```python
from build123d import *

# Parameters (mm, degrees)
F1_DEPTH = 38
F3_DEPTH = 25


with BuildPart() as f1:
    # F0 (on Right) → F1 (new body)
    with BuildSketch(Plane.YZ):
        Polygon((15, 19), (15, 20), (15, 24), (11, 24), (11, 15), (11, 6), (15, 6), (15, 10), (15, 11), (21.5, 11), (21.5, 8), (23.5, 8), (23.5, 15), (23.5, 22), (21.5, 22), (21.5, 19), align=None)
    extrude(amount=F1_DEPTH)

    # F2 (on face) → F3 (cut)
    with BuildSketch(Plane(origin=(0, 23.5, 0), x_dir=(-1, 0, 0), z_dir=(0, 1, 0))):
        with BuildLine():
            ThreePointArc((-17.35, 15), (-17.833274, 16.166726), (-19, 16.65))
            Line((-19, 16.65), (-19, 13.35))
            ThreePointArc((-19, 13.35), (-17.833274, 13.833274), (-17.35, 15))
        make_face()
        with BuildLine():
            Line((-19, 13.35), (-19, 16.65))
            ThreePointArc((-19, 16.65), (-20.65, 15), (-19, 13.35))
        make_face()
    extrude(amount=-F3_DEPTH, mode=Mode.SUBTRACT)


solid = f1.part
```
Read the model definition and answer for the solid it produces. Units are mm, in the model's axes. A direction names the side the tool comes from. Round coordinates to 2 decimals unless told otherwise and drop trailing zeros. Write each loop counter-clockwise with the first axis right and the second up, starting at its lowest first coordinate (ties: lowest second). Pieces come first, ordered by that corner, then holes. Notation, with made-up numbers: (5, 70.25) -> (39, 70.25) arc R20 cw to (39, 78.25) -> close; hole circle Ø2 at (-11.75, 9.25). An arc over 180 degrees is marked (long way). Answer in a Markdown table with one row per item. Add a question column.
1) Given P1, Ø3, axis at x = 19.5, y = 19.5, coming from the +Z side; P2, Ø0.6, axis at x = 14.5, y = 22.5, coming from the +Z side; P3, Ø0.6, axis at x = 13, y = 22.5, coming from the -Z side; P4, Ø7, axis at x = 23, y = 17, coming from the -Z side, each flat-ended and moving along its own axis, determine where each tip first touches the part or whether it passes through.
2) Find section B-B, the plane y = 20.5. Determine the outline of the cut face in (x, z).
3) Find section A-A, the plane z = 20.25. Determine the outline of the cut face in (x, y), and give its area (3 significant figures).
4) Find section C-C, the plane x = 34. Determine the outline of the cut face in (y, z), and give its area (3 significant figures).
5) Find section D-D, the plane z = 7.25. Determine the outline of the cut face in (x, y), and give its area (3 significant figures).
6) Determine the mould class of faces 1 (the face through (19, 11, 13)), 2 (the face through (19, 13, 24)), 3 (the face through (19, 15, 8)), 4 (the face through (19, 21.5, 10)) for opening direction Y: pulls with the +Y half, pulls with the -Y half, needs draft (parallel to the pull), parting line crosses it, or undercut.
7) Consider line 1 (Y direction, x = 8, z = 20.75); line 2 (Z direction, x = 35, y = 17.5); line 3 (Z direction, x = 17.5, y = 17.75). Determine where each line is inside the solid, lowest interval first.
8) Which of the six approach directions +Z, -Z, +X, -X, +Y, -Y give full straight-line access (tool end or side, diameter ignored) to faces 5 (the face through (19, 22, 8)), 6 (the face through (19, 18, 19)), 7 (the face through (19, 23, 22)), 8 (the face through (19, 18, 11))?
Findings below:
| question | item | result |
|---|---|---|
| 1 | P1 | z = 19 |
| 1 | P2 | z = 22 |
| 1 | P3 | z = 8 |
| 1 | P4 | z = 6 |
| 2 | outline | (0, 11) -> (38, 11) -> (38, 19) -> (0, 19) -> close; hole circle Ø3.3 at (19, 15) |
| 3 | outline | (0, 11) -> (38, 11) -> (38, 15) -> (0, 15) -> close; (0, 21.5) -> (38, 21.5) -> (38, 23.5) -> (0, 23.5) -> close |
| 3 | area | 228 mm² |
| 4 | outline | (11, 6) -> (15, 6) -> (15, 11) -> (21.5, 11) -> (21.5, 8) -> (23.5, 8) -> (23.5, 22) -> (21.5, 22) -> (21.5, 19) -> (15, 19) -> (15, 24) -> (11, 24) -> close |
| 4 | area | 152 mm² |
| 5 | outline | (0, 11) -> (38, 11) -> (38, 15) -> (0, 15) -> close |
| 5 | area | 152 mm² |
| 6 | face 1 | pulls with the -Y half |
| 6 | face 2 | needs draft |
| 6 | face 3 | undercut |
| 6 | face 4 | undercut |
| 7 | line 1 | 11 to 15, 21.5 to 23.5 |
| 7 | line 2 | 11 to 19 |
| 7 | line 3 | 11 to 14.31, 15.69 to 19 |
| 8 | face 5 | -Z, +X, -X, +Y |
| 8 | face 6 | +Z, +X, -X |
| 8 | face 7 | +Z, +X, -X, +Y |
| 8 | face 8 | -Z, +X, -X |
